The listing builds one solid part. Answer for the finished solid, in the listing's coordinates (mm). A direction names the side the tool comes from. Coordinates: 2 decimals unless noted, no trailing zeros. Order: outer loops, then holes, each group sorted by start corner. A loop starts at its lowest first (then second) coordinate and runs counter-clockwise, first axis right, second up.
from build123d import *

# Parameters (mm, degrees)
SKETCH1_R           = 75
BOSS_EXTRUDE1_DEPTH = 20
SKETCH2_R           = 60
BOSS_EXTRUDE2_DEPTH = 10
SKETCH3_R           = 75
BOSS_EXTRUDE3_DEPTH = 20
SKETCH4_R           = 30
BOSS_EXTRUDE4_DEPTH = 100
SKETCH5_R           = 100
BOSS_EXTRUDE5_DEPTH = 150
SKETCH6_R           = 80
BOSS_EXTRUDE6_DEPTH = 70
SKETCH7_R           = 10
BOSS_EXTRUDE7_DEPTH = 40
SKETCH13_R          = 25
CUT_EXTRUDE1_DEPTH  = 120
SKETCH14_R          = 10
BOSS_EXTRUDE8_DEPTH = 10


with BuildPart() as part:
    # Sketch1 → Boss-Extrude1 (new body)
    with BuildSketch(Plane(origin=(0, 0, 0), x_dir=(1, 0, 0), z_dir=(0, 1, 0))):
        with Locations(Location((0, 0, 0), (0, 0, 270))):
            Circle(SKETCH1_R)
    extrude(amount=BOSS_EXTRUDE1_DEPTH)

    # Sketch2 → Boss-Extrude2 (add)
    with BuildSketch(Plane(origin=(0, 20, 0), x_dir=(1, 0, 0), z_dir=(0, 1, 0))):
        with Locations(Location((0, 0, 0), (0, 0, 270))):
            Circle(SKETCH2_R)
    extrude(amount=BOSS_EXTRUDE2_DEPTH)

    # Sketch3 → Boss-Extrude3 (add)
    with BuildSketch(Plane(origin=(0, 30, 0), x_dir=(1, 0, 0), z_dir=(0, 1, 0))):
        with Locations(Location((0, 0, 0), (0, 0, 270))):
            Circle(SKETCH3_R)
    extrude(amount=BOSS_EXTRUDE3_DEPTH)

    # Sketch4 → Boss-Extrude4 (add)
    with BuildSketch(Plane(origin=(0, 50, 0), x_dir=(1, 0, 0), z_dir=(0, 1, 0))):
        with Locations(Location((0, 0, 0), (0, 0, 270))):
            Circle(SKETCH4_R)
    extrude(amount=BOSS_EXTRUDE4_DEPTH)

    # Sketch5 → Boss-Extrude5 (add)
    with BuildSketch(Plane(origin=(0, 0, 0), x_dir=(0, 0, -1), z_dir=(1, 0, 0))):
        with Locations((0, 154.201763101)):
            Circle(SKETCH5_R)
    extrude(amount=-BOSS_EXTRUDE5_DEPTH)

    # Sketch6 → Boss-Extrude6 (add)
    with BuildSketch(Plane(origin=(0, 0, 0), x_dir=(0, 0, -1), z_dir=(1, 0, 0))):
        with Locations(Location((0, 154.201763101, 0), (0, 0, 247.975687163))):
            Circle(SKETCH6_R)
    extrude(amount=BOSS_EXTRUDE6_DEPTH)

    # Sketch7 → Boss-Extrude7 (add)
    with BuildSketch(Plane(origin=(0, 0, 0), x_dir=(-1, 0, 0), z_dir=(0, -1, 0))):
        with Locations(Location((0, 50, 0), (0, 0, 270))):
            Circle(SKETCH7_R)
        with Locations(Location((-50, 0, 0), (0, 0, 270))):
            Circle(SKETCH7_R)
        with Locations(Location((0, -50, 0), (0, 0, 270))):
            Circle(SKETCH7_R)
        with Locations(Location((50, 0, 0), (0, 0, 270))):
            Circle(SKETCH7_R)
    extrude(amount=BOSS_EXTRUDE7_DEPTH)

    # Sketch13 → Cut-Extrude1 (cut)
    with BuildSketch(Plane(origin=(0, 0, 0), x_dir=(-1, 0, 0), z_dir=(0, -1, 0))):
        with Locations(Location((0, 0, 0), (0, 0, 90))):
            Circle(SKETCH13_R)
    extrude(amount=-CUT_EXTRUDE1_DEPTH, mode=Mode.SUBTRACT)

    # Sketch14 → Boss-Extrude8 (add)
    with BuildSketch(Plane(origin=(0, -40, 0), x_dir=(-1, 0, 0), z_dir=(0, -1, 0))):
        with Locations(Location((0, 50, 0), (0, 0, 270))):
            Circle(SKETCH14_R)
        with Locations(Location((50, 0, 0), (0, 0, 270))):
            Circle(SKETCH14_R)
        with Locations(Location((0, -50, 0), (0, 0, 270))):
            Circle(SKETCH14_R)
        with Locations(Location((-50, 0, 0), (0, 0, 270))):
            Circle(SKETCH14_R)
    extrude(amount=BOSS_EXTRUDE8_DEPTH)


solid = part.part
1) Determine the mould class of faces 1 (the face through (50, -50, 0)), 2 (the face through (-40.24, -24.65, -2.17)), 3 (the face through (0, -25, -60)), 4 (the face through (59.76, -24.65, -2.17)) for opening direction X: released by +X, released by -X, zero draft, split by the parting line, or undercut.
2) A tool of negligible diameter and unlimited length cuts with its end or side. For faces 5 (the face through (-32, 50, -1)), 6 (the face through (18, 0, -18)), 7 (the face through (-50, -50, 0)), 8 (the face through (0, 229, 30)), 9 (the face through (70, 155, -1)), from which of +Z, -Z, +X, -X, +Y, -Y can it reach the whole face along a straight path? Write none if from no direction.
3) Each of these flat-tipped pins is pushed along its axis until it touches: P1, Ø2, axis at x = 43.5, z = 52.5, coming from the -Y side; P2, Ø3, axis at x = 34, z = 33.5, coming from the +Y side; P3, Ø1, axis at y = 169.5, z = 52.5, coming from the +X side. Where does it stop, or does it pass through?
4) Consider L1, parallel to Y at x = 49.5, z = -53; L2, parallel to Y at x = -19.5, z = 64.5; L3, parallel to X at y = 29.5, z = 0. Determine where each line is inside the solid, lowest interval first.
5) Section A-A (z = -46.5) is taken. Give the vertices of the cut face in (x, y).
6) Section C-C (y = 130.5) is taken. Give the vertices of the cut face in (x, z), then the cut area to 3 significant figures.
7) Section B-B (x = 50) is taken. Give the vertices of the cut face in (y, z), then the cut area to 3 significant figures.
Filled sheet:
1. face 1: zero draft
1. face 2: undercut
1. face 3: split by the parting line
1. face 4: undercut
2. face 5: none
2. face 6: -Y
2. face 7: +Z, -Z, +X, -X, -Y
2. face 8: +X
2. face 9: +Z, -Z, +X, +Y
3. P1: stops at y = 0
3. P2: stops at y = 227.52
3. P3: stops at x = 70
4. L1: y = 0 to 20, 30 to 50, 94.28 to 214.13
4. L2: y = 0 to 20, 30 to 50, 77.78 to 230.62
4. L3: x = -60 to -25, 25 to 60
5. outline: (-150, 65.67) - (0, 65.67) - (0, 89.1) - (70, 89.1) - (70, 219.3) - (0, 219.3) - (0, 242.73) - (-150, 242.73) - close; (-58.85, 0) - (-9.37, 0) - (-9.37, -50) - (9.37, -50) - (9.37, 0) - (58.85, 0) - (58.85, 20) - (37.92, 20) - (37.92, 30) - (58.85, 30) - (58.85, 50) - (-58.85, 50) - (-58.85, 30) - (-37.92, 30) - (-37.92, 20) - (-58.85, 20) - close
6. outline: (-150, -97.15) - (0, -97.15) - (0, -76.41) - (70, -76.41) - (70, 76.41) - (0, 76.41) - (0, 97.15) - (-150, 97.15) - close
6. area: 39,800 mm2
7. outline: (-50, -10) - (0, -10) - (0, -55.9) - (20, -55.9) - (20, -33.17) - (30, -33.17) - (30, -55.9) - (50, -55.9) - (50, 55.9) - (30, 55.9) - (30, 33.17) - (20, 33.17) - (20, 55.9) - (0, 55.9) - (0, 10) - (-50, 10) - close; circle Ø160 at (154.2, 0)
7. area: 26,200 mm2
